Geometry check sheet. Reference: the model listing, model coordinates, mm. A direction names the side the tool comes from. Coordinates: 2 decimals unless noted, no trailing zeros. Order: outer loops, then holes, each group sorted by start corner. A loop starts at its lowest first (then second) coordinate and runs counter-clockwise, first axis right, second up. Notation, with made-up numbers: (-15.75, 81.25) -> (2.25, 81.25) arc R20 cw to (2.25, 102.25) -> close; hole circle Ø9 at (43.25, 34.5). An arc over 180 degrees is marked (long way). Answer in a Markdown table with one row per item. Add a question column.
Autodesk Inventor part; units mm, degrees
ref_plane "YZ Plane" through (0, 0, 0) normal (1, 0, 0) x (0, 1, 0)
ref_plane "XZ Plane" through (0, 0, 0) normal (0, 1, 0) x (-1, 0, 0)
ref_plane "XY Plane" through (0, 0, 0) normal (0, 0, 1) x (1, 0, 0)
sketch "Sketch1" plane through (0, 0, 0) normal (0, 1, 0) x (-1, 0, 0)
  line L0 (0, 0) -> (56, 0)
  line L1 (56, 0) -> (56, -85)
  line L2 (56, -85) -> (0, -85)
  line L3 (0, -85) -> (0, 0)
  line L4 (61, -90) -> (61, 5)
  line L5 (61, 5) -> (-5, 5)
  line L6 (-5, 5) -> (-5, -90)
  line L7 (61, -85) -> (-5, -85)
  dimension "d0" = 56
  dimension "d1" = 85
  dimension "d2" = 5
  dimension "d50" = 90
extrude "Extrusion1" add sketch "Sketch1" along normal blind 1
sketch "Sketch2" plane through (0, 1, 0) normal (0, 1, 0) x (1, 0, 0)
  line L0 (-61, -5) -> (5, -5)
  line L1 (-61, 85) -> (-61, -5)
  line L2 (-61, -5) -> (5, -5)
  line L3 (5, -5) -> (5, 85)
  line L4 (5, 85) -> (-61, 85)
  line L5 (-62, 86) -> (6, 86)
  line L6 (6, 86) -> (6, -6)
  line L7 (6, -6) -> (-62, -6)
  line L8 (-62, -6) -> (-62, 86)
  point P0 (0, 0)
  dimension "d41" = 1
sketch "Sketch4" plane through (0, 1, 0) normal (0, 1, 0) x (1, 0, 0)
  line L0 (0, 0) -> (-56, 0)
  line L1 (-56, 0) -> (-56, 85)
  line L2 (-56, 85) -> (0, 85)
  line L3 (0, 85) -> (0, 0)
  circle A0 centre (-3.5, 3.5) radius 1.375
  circle A1 centre (-52.5, 3.5) radius 1.375
  circle A2 centre (-52.5, 61.5) radius 1.375
  circle A3 centre (-3.5, 61.5) radius 1.375
  circle A4 centre (-52.5, 3.5) radius 3.1
  circle A5 centre (-52.5, 61.5) radius 3.1
  circle A6 centre (-3.5, 3.5) radius 3.1
  circle A7 centre (-3.5, 61.5) radius 3.1
  dimension "d14" = 56
  dimension "d15" = 85
  dimension "d16" = 2.75
  dimension "d17" = 2.75
  dimension "d18" = 2.75
  dimension "d19" = 2.75
  dimension "d20" = 49
  dimension "d21" = 58
  dimension "d22" = 58
  dimension "d23" = 49
  dimension "d24" = 6.2
  dimension "d25" = 6.2
  dimension "d26" = 6.2
  dimension "d27" = 6.2
  dimension "d28" = 3.5
  dimension "d29" = 3.5
  dimension "d30" = 3.5
  dimension "d31" = 3.5
  dimension "d32" = 3.5
hole "Hole1" at (-52.5, 1, -61.5) at (-52.5, 1, -3.5) at (-3.5, 1, -3.5) at (-3.5, 1, -61.5) direction (0, -1, 0) diameter 2.75 end through all
extrude "Extrusion4" add sketch "Sketch2" along normal blind 20 and the other way blind 1
sketch "Sketch5" plane through (6, 21, -86) normal (0, 0, -1) x (-1, 0, 0)
  line L0 (67, -20) -> (1, -20)
  line L1 (68, 0) -> (0, 0)
  line L2 (3, -20) -> (65, -20)
  line L3 (65, -20) -> (65, 0)
  line L4 (65, 0) -> (3, 0)
  line L5 (3, 0) -> (3, -20)
  line L6 (67, 0) -> (67, -20)
  line L7 (1, 0) -> (1, -20)
  point P0 (6, -21)
  dimension "d46" = 2
  dimension "d47" = 2
extrude "Extrusion5" cut sketch "Sketch5" against normal blind 2 contours L0 L5 L1 L3
sketch "Sketch6" plane through (6, 0, -86) normal (1, 0, 0) x (0, 0, -1)
  line L0 (0, 21) -> (0, 0)
  line L1 (-92, 21) -> (0, 21)
  line L2 (-92, 21) -> (-92, 0)
  line L3 (0, 0) -> (-92, 0)
  point P0 (-86, 0)
extrude "Extrusion6" add sketch "Sketch6" along normal blind 0.5
sketch "Sketch7" plane through (-62, 0, 6) normal (-1, 0, 0) x (0, 0, 1)
  line L0 (0, 21) -> (0, 0)
  line L1 (-92, 21) -> (0, 21)
  line L2 (-92, 0) -> (-92, 21)
  line L3 (0, 0) -> (-92, 0)
  point P0 (-6, 0)
extrude "Extrusion7" add sketch "Sketch7" along normal blind 0.5
sketch "Sketch8" plane through (0, 21, 0) normal (0, 1, 0) x (1, 0, 0)
  line L0 (6.5, -6) -> (-62.5, -6)
  line L1 (6.5, 86) -> (6.5, -6)
  line L2 (-62.5, -6) -> (-62.5, 86)
  line L3 (-59, 86) -> (3, 86)
  line L4 (-59, 86) -> (-62.5, 86)
  line L5 (3, 86) -> (6.5, 86)
  point P0 (0, 0)
  dimension "d55" = 92
  dimension "d56" = 69
sketch "Sketch9" plane through (-61, 1, 5) normal (1, 0, 0) x (0, 0, -1)
  line L0 (0, 0) -> (0, 20)
  line L1 (90, 20) -> (90, 0)
  line L2 (0, 20) -> (90, 20)
  line L3 (30, 16) -> (60, 16)
  line L4 (60, 16) -> (60, 15)
  line L5 (60, 15) -> (30, 15)
  line L6 (30, 15) -> (30, 16)
  point P0 (5, -1)
  point P1 (0, 16)
  point P2 (90, 15)
  dimension "d62" = 4
  dimension "d63" = 1
  dimension "d64" = 30
  dimension "d65" = 30
  dimension "d66" = 30
extrude "Extrusion8" cut sketch "Sketch9" against normal blind 1
ref_plane "Work Plane2" through (-28, 0, -86) normal (1, 0, 0) x (0, 0, -1)
mirror "Mirror1" about plane through (-28, 0, -86) normal (1, 0, 0) of "Extrusion8"
equation "\"d22\" = d21"
equation "\"d23\" = d20"
properties part number "bottom1"
(1) Cross-section at D-D (y = 3.25). Enter the section's corners in (x, z).
(2) Mould release check, pull along X, two halves, no side actions. Record for faces 1 (the face through (-28, 0, -39)), 2 (the face through (5, 11, -39)), 3 (the face through (-62.5, 11, -41)): +X half, -X half, draft (parallel to the pull), parting line (faces both ways), or undercut.
(3) Go/stop test with flat-tipped pins: P1, Ø10, axis at x = -22.5, y = 9.5, coming from the -Z side; P2, Ø4.5, axis at x = -52.5, z = -61.5, coming from the +Y side. Record where each tip stops, or that it passes through.
(4) Cross-section at B-B (x = -3.5). Enter the section's corners in (y, z) (3 decimals).
(5) Cross-section at A-A (z = -61.5). Enter the section's corners in (x, y) (3 decimals), plus the area to 4 significant figures.
(6) Scan lines: line 1 along Z through (x, y) = (-52.5, 0.35) (3 decimals); line 2 along X through (y, z) = (0.85, -3.5) (3 decimals); line 3 along X through (y, z) = (1.5, -48). Record each from-to range of solid material in increasing order.
(7) Cross-section at C-C (z = -33). Enter the section's corners in (x, y), plus the area to 3 significant figures.
(8) Access from +Z, -Z, +X, -X, +Y, -Y to the whole of each face (thin tool, end or side, straight path). Record for faces 4 (the face through (-2.97, 0.49, -60.23)), 5 (the face through (4, 11, -85)).
Checks:
| question | item | result |
|---|---|---|
| 1 | outline | (-62.5, -86) -> (-59, -86) -> (-59, -85) -> (-61, -85) -> (-61, 5) -> (5, 5) -> (5, -85) -> (3, -85) -> (3, -86) -> (6.5, -86) -> (6.5, 6) -> (-62.5, 6) -> close |
| 2 | face 1 | draft |
| 2 | face 2 | undercut |
| 2 | face 3 | -X half |
| 3 | P1 | z = 5 |
| 3 | P2 | y = 1 |
| 4 | outline | (0, -86) -> (1, -86) -> (1, -62.875) -> (0, -62.875) -> close; (0, -60.125) -> (1, -60.125) -> (1, -4.875) -> (0, -4.875) -> close; (0, -2.125) -> (1, -2.125) -> (1, 5) -> (21, 5) -> (21, 6) -> (0, 6) -> close |
| 5 | outline | (-62.5, 0) -> (-53.875, 0) -> (-53.875, 1) -> (-61, 1) -> (-61, 21) -> (-62.5, 21) -> close; (-51.125, 0) -> (-4.875, 0) -> (-4.875, 1) -> (-51.125, 1) -> close; (-2.125, 0) -> (6.5, 0) -> (6.5, 21) -> (5, 21) -> (5, 1) -> (-2.125, 1) -> close |
| 5 | area | 123.5 mm² |
| 6 | line 1 | -86 to -62.875, -60.125 to -4.875, -2.125 to 6 |
| 6 | line 2 | -62.5 to -53.875, -51.125 to -4.875, -2.125 to 6.5 |
| 6 | line 3 | -62.5 to -61, 5 to 6.5 |
| 7 | outline | (-62.5, 0) -> (6.5, 0) -> (6.5, 21) -> (5, 21) -> (5, 17) -> (6, 17) -> (6, 16) -> (5, 16) -> (5, 1) -> (-61, 1) -> (-61, 16) -> (-62, 16) -> (-62, 17) -> (-61, 17) -> (-61, 21) -> (-62.5, 21) -> close |
| 7 | area | 127 mm² |
| 8 | face 4 | +Y, -Y |
| 8 | face 5 | +Y |
